The drawing under review shows one solid part. Ordinate dimensions are in mm from its lowest x, y, z. A direction names the side the tool comes from. Coordinates: 2 decimals unless noted, no trailing zeros. Write each loop counter-clockwise with the first axis right and the second up, starting at its lowest first coordinate (ties: lowest second). Pieces come first, ordered by that corner, then holes. Notation, with made-up numbers: (-24.75, -25) - (32.25, -25) arc R22 ccw to (32.25, -19) - close; hole circle Ø11 at (48.5, 7.5). An arc over 180 degrees is marked (long way). Answer as CSV lines item,"result". Start each with the question number.
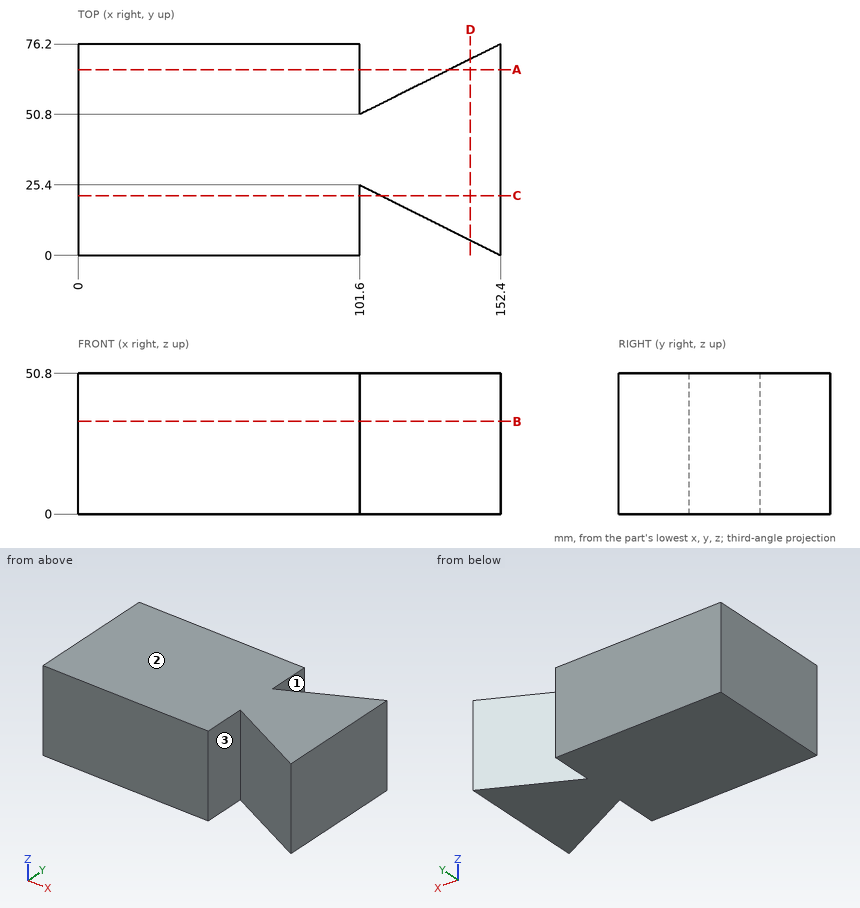
(1) For the marked faces 1, 2 and 3, list the 3-axis set-ups (+Z, -Z, +X, -X, +Y, -Y) from which the entire face can be reached by the end or side of a thin tool; tool diameter is ignored.
(2) Wall thickness on line 1 (X direction, y = 63, z = 43); line 2 (X direction, y = 58.5, z = 25.5); line 3 (Y direction, x = 118.5, z = 6): over which ranges is each line inside the solid? List them lowest first.
(3) Add section D-D on x = 141.5. Give the boundary of the cut face in (y, z).
(4) For pin 1 (2 mm diameter, centred on x = 112.5, z = 43.5, fed in from -Y); pin 2 (8 mm diameter, centred on x = 116, z = 39, fed in from +Y); pin 3 (5 mm diameter, centred on x = 116.5, z = 22.5, fed in from +Y), all flat-tipped, find the tip position at first contact; note any pin that passes through.
(5) Add section C-C on y = 21.5. Give the boundary of the cut face in (x, z).
(6) Add section B-B on z = 33.5. Give the boundary of the cut face in (x, y).
(7) Add section A-A on y = 67. Give the boundary of the cut face in (x, z), then the cut area to 3 significant figures.
Reported:
1,face 1,"+Z, -Z, +Y"
1,face 2,"+Z, +X, -X, +Y, -Y"
1,face 3,"+Z, -Z, -Y"
2,line 1,"0 to 101.6, 126 to 152.4"
2,line 2,"0 to 101.6, 117 to 152.4"
2,line 3,"16.95 to 59.25"
3,outline,"(5.45, 0) - (70.75, 0) - (70.75, 50.8) - (5.45, 50.8) - close"
4,pin 1,"y = 19.45"
4,pin 2,"y = 60"
4,pin 3,"y = 59.5"
5,outline,"(0, 0) - (101.6, 0) - (101.6, 50.8) - (0, 50.8) - close; (109.4, 0) - (152.4, 0) - (152.4, 50.8) - (109.4, 50.8) - close"
6,outline,"(0, 0) - (101.6, 0) - (101.6, 25.4) - (152.4, 0) - (152.4, 76.2) - (101.6, 50.8) - (101.6, 76.2) - (0, 76.2) - close"
7,outline,"(0, 0) - (101.6, 0) - (101.6, 50.8) - (0, 50.8) - close; (134, 0) - (152.4, 0) - (152.4, 50.8) - (134, 50.8) - close"
7,area,"6,100 mm²"
